Autodesk Inventor part; units mm, degrees
ref_plane "YZ Plane" through (0, 0, 0) normal (1, 0, 0) x (0, 1, 0)
ref_plane "XZ Plane" through (0, 0, 0) normal (0, 1, 0) x (-1, 0, 0)
ref_plane "XY Plane" through (0, 0, 0) normal (0, 0, 1) x (1, 0, 0)
sketch "Sketch1" plane through (0, 0, 0) normal (0, 1, 0) x (-1, 0, 0)
  line L0 (0, 0) -> (-304.8, 0)
  line L1 (-304.8, 0) -> (-304.8, -84.8294)
  line L2 (-304.8, -84.8294) -> (0, -84.8294)
  line L3 (0, -84.8294) -> (0, 0)
  dimension "d0" = 304.8
extrude "Extrusion1" add sketch "Sketch1" along normal blind 3.175
sketch "Sketch2" plane through (0, 3.175, 0) normal (0, 1, 0) x (1, 0, 0)
  line L0 (0, 0) -> (304.8, 0)
  line L1 (3.175, 0) -> (3.175, 81.6544)
  line L2 (3.175, 81.6544) -> (301.625, 81.6544)
  line L3 (301.625, 81.6544) -> (301.625, 0)
  line L4 (304.8, 0) -> (304.8, 84.8294)
  line L5 (0, 84.8294) -> (0, 0)
  line L6 (304.8, 84.8294) -> (0, 84.8294)
  line L7 (0, 0) -> (3.175, 0)
  line L8 (304.8, 0) -> (301.625, 0)
  dimension "d3" = 3.175
  dimension "d4" = 3.175
  dimension "d5" = 3.175
extrude "Extrusion2" add sketch "Sketch2" along normal blind 152.4 contours L5 L6 L4 L0 L3 L2 L1
sketch "Sketch4" plane through (3.175, 3.175, -81.6544) normal (0, 0, 1) x (1, 0, 0)
  line L0 (-3.175, 152.4) -> (73.025, 228.6)
  line L1 (301.625, 152.4) -> (-3.175, 152.4)
  line L2 (301.625, 152.4) -> (225.425, 228.6)
  line L3 (225.425, 228.6) -> (73.025, 228.6)
  point P0 (-3.175, -3.175)
  point P1 (-3.175, 152.4)
  dimension "d11" = 152.4
  dimension "d12" = 76.2
extrude "Extrusion3" add sketch "Sketch4" against normal blind 3.175
sketch "Sketch7" plane through (3.175, 3.175, -81.6544) normal (0, 0, 1) x (1, 0, 0)
  line L0 (0.6738, 152.4) -> (76.8738, 228.6)
  line L1 (-3.175, 152.4) -> (73.025, 228.6)
  line L2 (0.6738, 152.4) -> (-3.175, 152.4)
  line L3 (73.025, 228.6) -> (225.425, 228.6)
  line L4 (73.025, 228.6) -> (76.8738, 228.6)
  point P0 (-3.175, -3.175)
extrude "Extrusion4" add sketch "Sketch7" along normal blind 82.042
sketch "Sketch8" plane through (3.175, 3.175, -81.6544) normal (0, 0, 1) x (1, 0, 0)
  line L0 (301.625, -3.175) -> (301.625, 152.4)
  line L1 (298.45, 0) -> (298.45, 152.4)
  line L2 (301.625, 152.4) -> (298.45, 152.4)
  line L3 (298.45, 152.4) -> (222.25, 228.6)
  line L4 (76.8738, 228.6) -> (225.425, 228.6)
  line L5 (301.625, 152.4) -> (225.425, 228.6)
  point P0 (-3.175, -3.175)
  dimension "d19" = 3.175
extrude "Extrusion5" add sketch "Sketch8" along normal blind 82.042
properties part number "15102898-16-P-0203"
Part model, mm, in its own coordinate system. A direction names the side the tool comes from. Round coordinates to 2 decimals unless told otherwise and drop trailing zeros. Order: outer loops, then holes, each group sorted by start corner. A loop starts at its lowest first (then second) coordinate and runs counter-clockwise, first axis right, second up. Notation, with made-up numbers: M 66,1.25 L 124,1.25 A3 cw 124,6.25 Z; hole C 88,-16.75 d6. An arc over 180 degrees is marked long. Answer in a Markdown table with one row per item. Add a question column.
Q1. Cut at D-D on x = 70. Give the cut face in (y, z) (3 decimals).
Q2. Cut at B-B on x = 172. Give the cut face in (y, z) (3 decimals), and give its area (3 significant figures).
Q3. Cut at C-C on z = -74. Give the cut face in (x, y) (3 decimals), and give its area (3 significant figures).
Q4. Cut at A-A on y = 88. Give the cut face in (x, z) (3 decimals), and give its area (3 significant figures).
Q5. Pin check, flat tips, straight feed: pin 1 (5 mm diameter, centred on x = 214, y = 170, fed in from +Z); pin 2 (6 mm diameter, centred on x = 98.5, z = -58, fed in from +Y) (3 decimals). Stop position of each tip, or through.
Q6. Mould opens along Y. For faces 1 (the face through (155, 0, -42)), 2 (the face through (301.625, 78, -41)), 3 (the face through (0, 77, -43)) say: +Y half, -Y half, draft (parallel to the pull), parting line (faces both ways), or undercut.
Q7. Wall check: L1, parallel to X at y = 73.5, z = -79.5 (3 decimals); L2, parallel to Z at x = 52, y = 124; L3, parallel to Y at x = 111, z = -52.5 (3 decimals). Give the ranges that are in metal, low to high. Write a range as from..to.
Q8. 3-axis set-ups, long thin cutter, end or side, ignore diameter. For faces 4 (the face through (152, 3, 0)), 5 (the face through (150, 118, -84.829)), 6 (the face through (150, 119, -81.654)): which of +Z, -Z, +X, -X, +Y, -Y reach the whole face in a straight line?
Established:
| question | item | result |
|---|---|---|
| 1 | outline | M 0,-84.829 L 225.575,-84.829 L 225.575,0.388 L 221.726,0.388 L 221.726,-81.654 L 3.175,-81.654 L 3.175,0 L 0,0 Z |
| 2 | outline | M 0,-84.829 L 231.775,-84.829 L 231.775,-81.654 L 3.175,-81.654 L 3.175,0 L 0,0 Z |
| 2 | area | 995 mm2 |
| 3 | outline | M 0,0 L 304.8,0 L 304.8,155.575 L 228.6,231.775 L 225.425,231.775 L 301.625,155.575 L 301.625,3.175 L 3.175,3.175 L 3.175,155.575 L 3.849,155.575 L 80.049,231.775 L 76.2,231.775 L 0,155.575 Z |
| 3 | area | 2,470 mm2 |
| 4 | outline | M 0,-84.829 L 304.8,-84.829 L 304.8,0 L 301.625,0 L 301.625,-81.654 L 3.175,-81.654 L 3.175,0 L 0,0 Z |
| 4 | area | 1,490 mm2 |
| 5 | pin 1 | stops at z = -81.65 |
| 5 | pin 2 | stops at y = 3.175 |
| 6 | face 1 | -Y half |
| 6 | face 2 | undercut |
| 6 | face 3 | draft |
| 7 | L1 | x = 0..3.175, 301.625..304.8 |
| 7 | L2 | z = -84.83..-81.65 |
| 7 | L3 | y = 0..3.175 |
| 8 | face 4 | +Z, +X, -X, -Y |
| 8 | face 5 | -Z, +X, -X, +Y, -Y |
| 8 | face 6 | +Z |
